The model under review builds one solid part; all positions refer to its coordinate system, in mm. A direction names the side the tool comes from. Round coordinates to 2 decimals unless told otherwise and drop trailing zeros. Order: outer loops, then holes, each group sorted by start corner. A loop starts at its lowest first (then second) coordinate and runs counter-clockwise, first axis right, second up.
1) To check wall thickness, follow L1, parallel to X at y = 1.25, z = -3; L2, parallel to X at y = 1, z = 0; L3, parallel to Y at x = 7, z = 2.75. State the ranges of each line that lie inside material, in increasing order.
2) Consider section C-C (y = -0.75). Give the boundary of the cut face in (x, z), then the cut area to 3 significant figures.
3) Consider section A-A (z = 0). Give the boundary of the cut face in (x, y), then the cut area to 3 significant figures.
4) Clearance check with flat-ended pins moving along their axes: P1, Ø3, axis at x = 14.5, y = 2, coming from the +Z side; P2, Ø2, axis at y = -2.5, z = 0.5, coming from the +X side. State where each tip first meets the part, or that it passes through.
5) Consider section D-D (z = 2). Give the boundary of the cut face in (x, y).
6) Machinability: for faces 1 (the face through (7.888, -1.341, -3.233)), 2 (the face through (-0.39, 1.01, 0.65)), which of the approach directions +Z, -Z, +X, -X, +Y, -Y give a long, thin tool a straight path to every point of the face, cutting with its end or side? Answer none if there is none.
7) Consider section B-B (x = 14). Give the boundary of the cut face in (y, z).
from build123d import *

# Parameters (mm, degrees)
SKETCH1_R           = 3.5
BOSS_EXTRUDE1_DEPTH = 16
SKETCH2_R           = 1.2
BOSS_EXTRUDE2_DEPTH = 0.8
SKETCH3_R           = 0.5
BOSS_EXTRUDE3_DEPTH = 4.2
SKETCH4_R           = 0.3
BOSS_EXTRUDE4_DEPTH = 1


with BuildPart() as part:
    # Sketch1 → Boss-Extrude1 (new body)
    with BuildSketch(Plane(origin=(0, 0, 0), x_dir=(0, 0, -1), z_dir=(1, 0, 0))):
        Circle(SKETCH1_R)
    extrude(amount=BOSS_EXTRUDE1_DEPTH)

    # Sketch2 → Boss-Extrude2 (add)
    with BuildSketch(Plane.ZY):
        Circle(SKETCH2_R)
    extrude(amount=BOSS_EXTRUDE2_DEPTH)

    # Sketch3 → Boss-Extrude3 (add)
    with BuildSketch(Plane.ZY.offset(0.8)):
        Circle(SKETCH3_R)
    extrude(amount=BOSS_EXTRUDE3_DEPTH)

    # Sketch4 → Boss-Extrude4 (add)
    with BuildSketch(Plane(origin=(16, 0, 0), x_dir=(0, 0, -1), z_dir=(1, 0, 0))):
        with Locations((-2, 0)):
            Circle(SKETCH4_R)
        with Locations((2, 0)):
            Circle(SKETCH4_R)
    extrude(amount=BOSS_EXTRUDE4_DEPTH)


solid = part.part
Answer below:
1. L1: x = 0 to 16
1. L2: x = -0.8 to 16
1. L3: y = -2.17 to 2.17
2. outline: (-0.8, -0.94) - (0, -0.94) - (0, -3.42) - (16, -3.42) - (16, 3.42) - (0, 3.42) - (0, 0.94) - (-0.8, 0.94) - close
2. area: 111 mm2
3. outline: (-5, -0.5) - (-0.8, -0.5) - (-0.8, -1.2) - (0, -1.2) - (0, -3.5) - (16, -3.5) - (16, 3.5) - (0, 3.5) - (0, 1.2) - (-0.8, 1.2) - (-0.8, 0.5) - (-5, 0.5) - close
3. area: 118 mm2
4. P1: stops at z = 3.46
4. P2: stops at x = 16
5. outline: (0, -2.87) - (16, -2.87) - (16, -0.3) - (17, -0.3) - (17, 0.3) - (16, 0.3) - (16, 2.87) - (0, 2.87) - close
6. face 1: +X, -X
6. face 2: -X
7. outline: circle Ø7 at (0, 0)
